Geometry: see drawing. Coordinates: mm, zero at the bounding-box minimum. A direction names the side the tool comes from. Give positions to 0.01 mm unless a question says otherwise; leave off trailing zeros. Write each loop counter-clockwise with the first axis right and the second up, starting at its lowest first coordinate (ties: lowest second). Pieces come first, ordered by that corner, then holes. Notation, with made-up numbers: M 14.25,-4 L 69.25,-4 A22 cw 69.25,14 Z; hole C 64,88.25 d3. An arc over 180 degrees is marked long. Use one line per item in the form item = value. Start each with the question number.
Item 1: Section query D-D on z = 5.25. Return loops of the section in (x, y), then the cut area to 3 significant figures.
Item 2: Section query B-B on y = 9.5. Return loops of the section in (x, z), then the cut area to 3 significant figures.
Item 3: Access query for the marked faces 1 and 2. Directions: +Z, -Z, +X, -X, +Y, -Y. A direction counts if a zero-diameter tool reaches every point of the face in a straight line with its end or side. Return the directions, or none.
Item 4: Section query A-A on x = 2.02. Return loops of the section in (y, z) (3 decimals), then the cut area to 3 significant figures.
Item 5: Pull-direction query (X, two-part tool) for the marked faces 3 and 4; classes: released by +X, released by -X, zero draft, split by the parting line, or undercut.
Item 6: Material intervals for line 1 along Y through (x, z) = (2.02, 0.3) (3 decimals); line 2 along X through (y, z) = (12.5, 5.3); line 3 along Z through (x, y) = (17, 12.5), sorted ascending. Write a range as from..to.
Item 7: Section query C-C on x = 21.75. Return loops of the section in (y, z), then the cut area to 3 significant figures.
Item 8: Contact query for flat-ended pins moving along their axis: P1, Ø12, axis at x = 17, y = 10.5, coming from the -Z side; P2, Ø2.5, axis at x = 27.5, z = 2.5, coming from the -Y side; P3, Ø1, axis at y = 12, z = 5, coming from the -X side; P4, Ø10, axis at x = 18, y = 6.5, coming from the +Z side. Output: stop coordinate, or through.
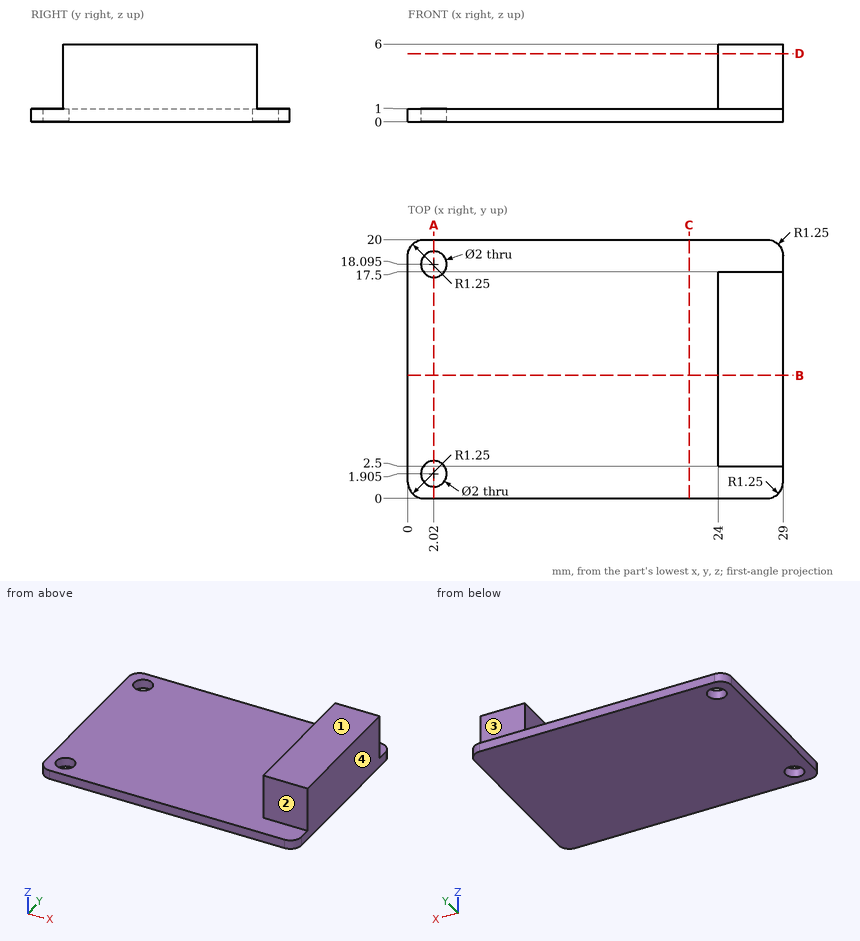
Answer sheet:
q1.outline = M 24,2.5 L 29,2.5 L 29,17.5 L 24,17.5 Z
q1.area = 75.0 mm2
q2.outline = M 0,0 L 29,0 L 29,6 L 24,6 L 24,1 L 0,1 Z
q2.area = 54.0 mm2
q3.face_1 = +Z, +X, -X, +Y, -Y
q3.face_2 = +Z, +X, -X, -Y
q4.outline = M 0,0 L 0.905,0 L 0.905,1 L 0,1 Z; M 2.905,0 L 17.095,0 L 17.095,1 L 2.905,1 Z; M 19.095,0 L 20,0 L 20,1 L 19.095,1 Z
q4.area = 16.0 mm2
q5.face_3 = zero draft
q5.face_4 = released by +X
q6.line_1 = 0..0.905, 2.905..17.095, 19.095..20
q6.line_2 = 24..29
q6.line_3 = 0..1
q7.outline = M 0,0 L 20,0 L 20,1 L 0,1 Z
q7.area = 20.0 mm2
q8.P1 = 0
q8.P2 = 2.5
q8.P3 = 24
q8.P4 = 1
